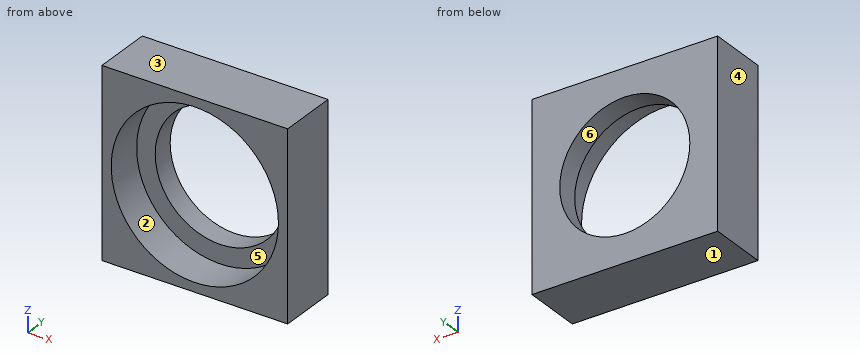
from build123d import *

# Parameters (mm, degrees)
SKETCH1_W           = 10
SKETCH1_H           = 10
SKETCH1_R           = 4.5
BOSS_EXTRUDE1_DEPTH = 3.175
SKETCH2_W           = 10
SKETCH2_H           = 10
SKETCH2_R           = 3.5
BOSS_EXTRUDE2_DEPTH = 1.175


with BuildPart() as part:
    # Sketch1 → Boss-Extrude1 (new body)
    with BuildSketch(Plane(origin=(0, 0, 0), x_dir=(1, 0, 0), z_dir=(0, 1, 0))):
        with Locations((5, -5)):
            Rectangle(SKETCH1_W, SKETCH1_H)
        with Locations((5, -5)):
            Circle(SKETCH1_R, mode=Mode.SUBTRACT)
    extrude(amount=BOSS_EXTRUDE1_DEPTH)

    # Sketch2 → Boss-Extrude2 (add)
    with BuildSketch(Plane(origin=(0, 3.175, 0), x_dir=(1, 0, 0), z_dir=(0, 1, 0))):
        with Locations((5, -5)):
            Rectangle(SKETCH2_W, SKETCH2_H)
        with Locations((5, -5)):
            Circle(SKETCH2_R, mode=Mode.SUBTRACT)
    extrude(amount=-BOSS_EXTRUDE2_DEPTH)


solid = part.part
Part model, mm, in its own coordinate system. Face numbers are marked on the shaded views. A direction names the side the tool comes from. Coordinates: 2 decimals unless noted, no trailing zeros. Loops run counter-clockwise (first coordinate to the right, second up) from the corner with the lowest first, then second, coordinate; pieces in that order, holes last. Notation, with made-up numbers: (-22.75, -37.5) -> (19.25, -37.5) arc R22 ccw to (19.25, -10.5) -> close; hole circle Ø5 at (-38.75, 7). An arc over 180 degrees is marked (long way). Use a Markdown table: item, result. Add a question column.
Item 1: Which spindle directions (+Z, -Z, +X, -X, +Y, -Y) get a long thin tool onto all of the face, cutting with end or side? Do the marked faces 1 and 2. Say none if no direction does.
Item 2: Band-saw the part on B-B on y = 1.15. Write the cut outline in (x, z), plus the area to 3 significant figures.
Item 3: Probe probe 1 along X at (y, z) = (2.9, 5); probe 2 along Z at (x, y) = (5, 0.7). List the from-to ranges inside material, lowest first.
Item 4: Band-saw the part on D-D on z = 1. Write the cut outline in (x, y) (3 decimals).
Item 5: Pull direction Z, two halves, no side cores. Call the marked faces 3, 4, 5 and 6: +Z half, -Z half, draft (parallel to the pull), parting line (faces both ways), or undercut.
Item 6: Band-saw the part on C-C on x = 8.25. Write the cut outline in (y, z) (3 decimals).
Item 7: Band-saw the part on A-A on z = 5. Write the cut outline in (x, y) (3 decimals), plus the area to 4 significant figures.
Geometry says:
| question | item | result |
|---|---|---|
| 1 | face 1 | -Z, +X, -X, +Y, -Y |
| 1 | face 2 | -Y |
| 2 | outline | (0, 0) -> (10, 0) -> (10, 10) -> (0, 10) -> close; hole circle Ø9 at (5, 5) |
| 2 | area | 36.4 mm² |
| 3 | probe 1 | 0 to 1.5, 8.5 to 10 |
| 3 | probe 2 | 0 to 0.5, 9.5 to 10 |
| 4 | outline | (0, 0) -> (2.938, 0) -> (2.938, 2) -> (7.062, 2) -> (7.062, 0) -> (10, 0) -> (10, 3.175) -> (0, 3.175) -> close |
| 5 | face 3 | +Z half |
| 5 | face 4 | draft |
| 5 | face 5 | undercut |
| 5 | face 6 | undercut |
| 6 | outline | (0, 0) -> (3.175, 0) -> (3.175, 3.701) -> (2, 3.701) -> (2, 1.888) -> (0, 1.888) -> close; (0, 8.112) -> (2, 8.112) -> (2, 6.299) -> (3.175, 6.299) -> (3.175, 10) -> (0, 10) -> close |
| 7 | outline | (0, 0) -> (0.5, 0) -> (0.5, 2) -> (1.5, 2) -> (1.5, 3.175) -> (0, 3.175) -> close; (8.5, 2) -> (9.5, 2) -> (9.5, 0) -> (10, 0) -> (10, 3.175) -> (8.5, 3.175) -> close |
| 7 | area | 5.525 mm² |
